Could you check a few things on this drawing? It's one solid part, dimensions in mm from its lowest x, y, z. Give positions to 0.01 mm unless a question says otherwise; leave off trailing zeros. Write each loop counter-clockwise with the first axis right and the second up, starting at its lowest first coordinate (ties: lowest second). Pieces come first, ordered by that corner, then holes. Notation, with made-up numbers: M 25,-17.5 L 61,-17.5 A13 ccw 61,-4.5 Z; hole C 13,-18.75 d9. An arc over 180 degrees is marked long. Answer as CSV lines item,"result". Start each with the question number.
Q1. Suppose I cut it at C-C (x = 92.71). Write out the boundary of the cut face in (y, z) (1 decimal).
Q2. If I drill on line 1 along X through (y, z) = (1.6, 79.5) (1 decimal); line 2 along X through (y, z) = (2.5, 5.5) (1 decimal); line 3 along Z through (x, y) = (18, 2.1) (1 decimal), over which ranges is the centre line in solid material (lowest first)?
Q3. Suppose I cut it at D-D (z = 57). Write out the boundary of the cut face in (x, y) (1 decimal).
Q4. Suppose I cut it at A-A (z = 39). Write out the boundary of the cut face in (x, y) (1 decimal).
Q5. For pin 1 (1 mm diameter, centred on x = 162, y = 1.5, fed in from +Z) (1 decimal); pin 2 (1.6 mm diameter, centred on x = 160.5, y = 1.5, fed in from -Z); pin 3 (1.5 mm diameter, centred on x = 70, y = 1, fed in from +Z), each with a flat end and sliding along its axis, tell me the tip position at first contact or that it passes through.
Q6. Suppose I cut it at B-B (y = 1.1). Write out the boundary of the cut face in (x, z), then the cut area to 3 significant figures.
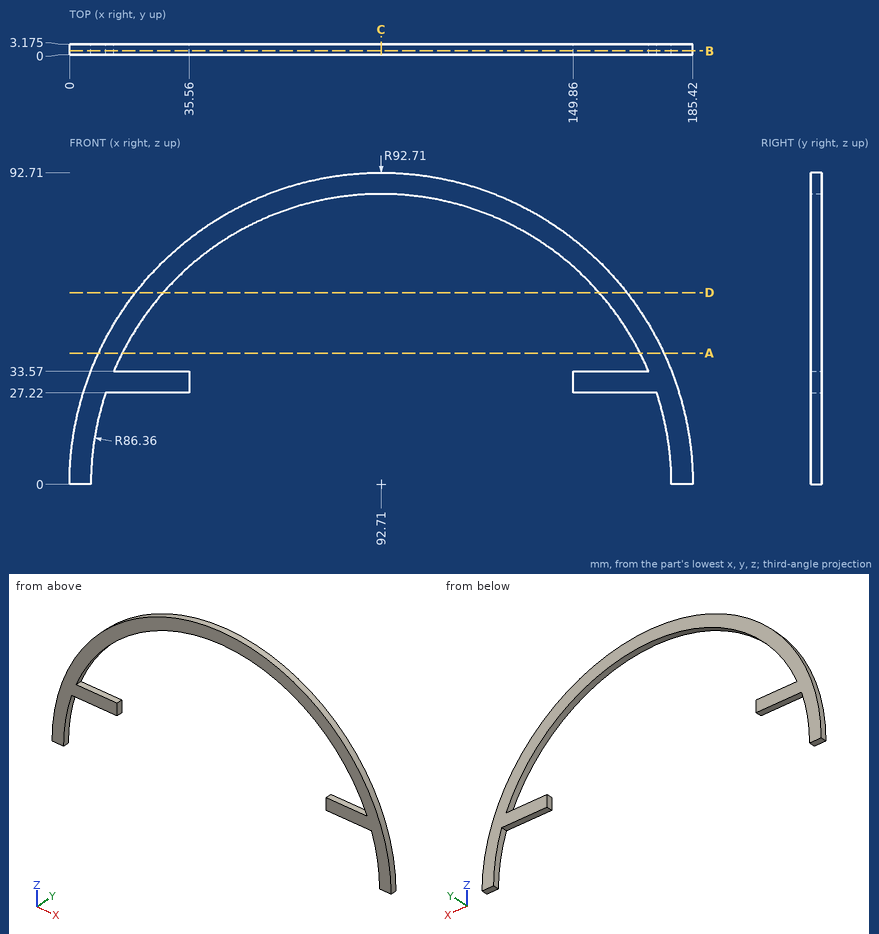
Resolved:
1,outline,"M 0,86.4 L 3.2,86.4 L 3.2,92.7 L 0,92.7 Z"
2,line 1,"45 to 59, 126.4 to 140.4"
2,line 2,"0.2 to 6.5, 178.9 to 185.3"
2,line 3,"27.2 to 33.6, 43.3 to 54.9"
3,outline,"M 19.6,0 L 27.8,0 L 27.8,3.2 L 19.6,3.2 Z; M 157.6,0 L 165.8,0 L 165.8,3.2 L 157.6,3.2 Z"
4,outline,"M 8.6,0 L 15.7,0 L 15.7,3.2 L 8.6,3.2 Z; M 169.8,0 L 176.8,0 L 176.8,3.2 L 169.8,3.2 Z"
5,pin 1,"z = 62.2"
5,pin 2,"z = 27.22"
5,pin 3,"z = 90.07"
6,outline,"M 0,0 L 6.35,0 A86.36 cw 10.75,27.22 L 35.56,27.22 L 35.56,33.57 L 13.14,33.57 A86.36 cw 172.28,33.57 L 149.86,33.57 L 149.86,27.22 L 174.67,27.22 A86.36 cw 179.07,0 L 185.42,0 A92.71 ccw Z"
6,area,"2,090 mm^2"
